Input: dimensioned drawing with shaded views. Units: mm. Origin: part minimum x, y, z. Give positions to 0.01 mm unless a question says otherwise; leave off trailing zeros. Loops run counter-clockwise (first coordinate to the right, second up) from the corner with the lowest first, then second, coordinate; pieces in that order, holes last. Notation, with made-up numbers: M 84.5,-20 L 119.5,-20 A31 ccw 119.5,16 Z; hole C 53.5,-2.75 d6. An arc over 180 degrees is marked long. Answer in a Markdown table with one row per item.
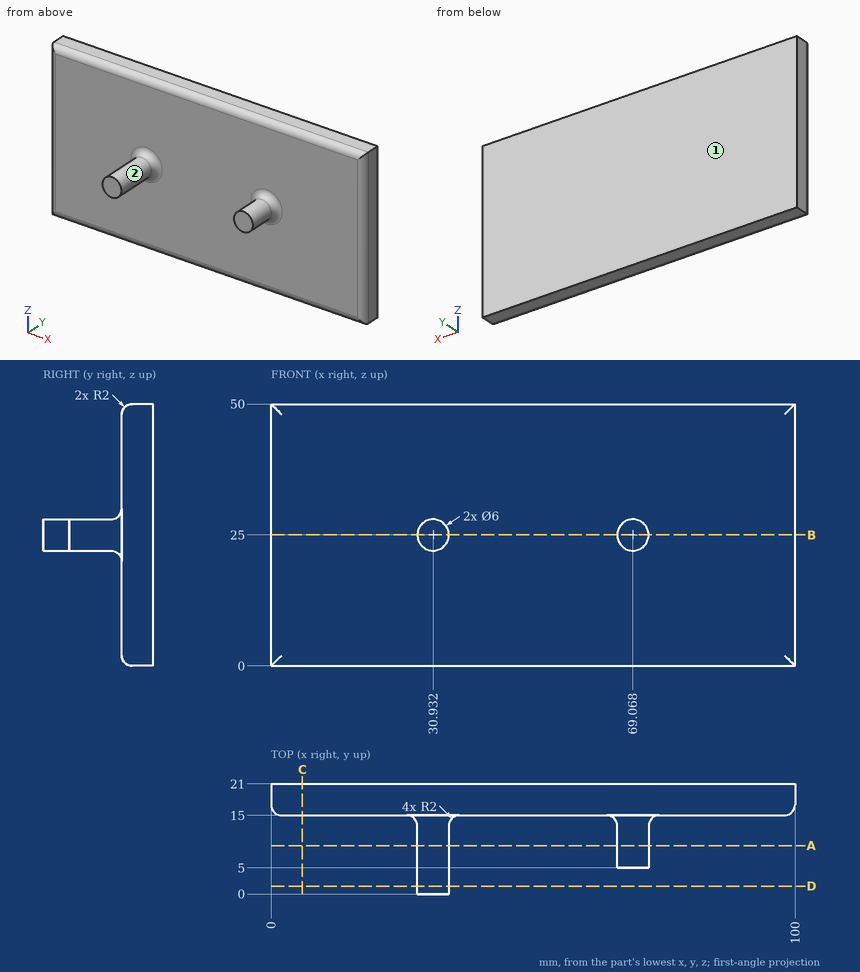
Q1. Section query B-B (z = 25). Output: boundary loops of the cut face in (x, y), plus the area to 3 significant figures.
Values follow:
| item | result |
|---|---|
| outline | M 0,17 A2 ccw 2,15 L 25.93,15 A2 cw 27.93,13 L 27.93,0 L 33.93,0 L 33.93,13 A2 cw 35.93,15 L 64.07,15 A2 cw 66.07,13 L 66.07,5 L 72.07,5 L 72.07,13 A2 cw 74.07,15 L 98,15 A2 ccw 100,17 L 100,21 L 0,21 Z |
| area | 752 mm^2 |
Q2. Section query A-A (y = 9.25). Output: boundary loops of the cut face in (x, z), plus the area to 3 significant figures.
Values follow:
| item | result |
|---|---|
| outline | C 30.93,25 d6; C 69.07,25 d6 |
| area | 56.5 mm^2 |
Q3. Ray query, probe 1 along Y at (x, z) = (16.5, 39.5); probe 2 along Z at (x, y) = (28.5, 4); probe 3 along Z at (x, y) = (67, 15.25). Return the intervals inside material, ascending. Write a range as from..to.
Values follow:
| item | result |
|---|---|
| probe 1 | 15..21 |
| probe 2 | 23.24..26.76 |
| probe 3 | 1.03..48.97 |
Q4. Section query C-C (x = 6). Output: boundary loops of the cut face in (y, z), plus the area to 3 significant figures.
Values follow:
| item | result |
|---|---|
| outline | M 15,2 A2 ccw 17,0 L 21,0 L 21,50 L 17,50 A2 ccw 15,48 Z |
| area | 298 mm^2 |
Q5. Contact query for flat-ended pins moving along their axis: pin 1 Ø3 at (y, z) = (6, 23.5) entering from +X; pin 2 Ø14 at (x, z) = (55, 26.5) entering from -Y; pin 3 Ø3 at (x, z) = (70.5, 25.5) entering from -Y. Output: stop coordinate, or through.
Values follow:
| item | result |
|---|---|
| pin 1 | x = 72.07 |
| pin 2 | y = 15 |
| pin 3 | y = 5 |
Q6. Section query D-D (y = 1.5). Output: boundary loops of the cut face in (x, z).
Values follow:
| item | result |
|---|---|
| outline | C 30.93,25 d6 |
Q7. Mould query, pull axis X, two halves, no side actions, for the marked faces 1 and 2. Classes: +X half, -X half, draft (parallel to the pull), parting line (faces both ways), or undercut.
Values follow:
| item | result |
|---|---|
| face 1 | draft |
| face 2 | undercut |
